Read the model definition and answer for the solid it produces. Units are mm, in the model's axes. A direction names the side the tool comes from. Coordinates: 2 decimals unless noted, no trailing zeros. Order: outer loops, then holes, each group sorted by start corner. A loop starts at its lowest first (then second) coordinate and runs counter-clockwise, first axis right, second up. Notation, with made-up numbers: (28, -4) -> (48, -4) arc R16 ccw to (48, 16) -> close; hole circle Ø6 at (1.5, -32). An arc over 180 degrees is marked (long way). Answer in a Markdown table with one row per item.
Autodesk Fusion 360 part; units mm, degrees
sketch "Sketch1" plane through (0, 0, 0) normal (0, 0, 1) x (1, 0, 0)
  line L0 (20, 20) -> (-20, 20)
  line L1 (-20, 20) -> (-20, -20)
  line L2 (-20, -20) -> (20, -20)
  line L3 (20, -20) -> (20, 20)
  line L4 (20, 20) -> (-20, -20) construction
  line L5 (-20, 20) -> (20, -20) construction
  dimension "d1" = 40
  dimension "d2" = 40
extrude "Extrude1" add sketch "Sketch1" along normal blind 8
sketch "Sketch2" plane through (0, 0, 8) normal (0, 0, 1) x (-1, 0, 0)
  line L0 (-20, 20) -> (-20, -20)
  line L1 (-20, -20) -> (20, -20)
  line L2 (20, -20) -> (20, 20)
  line L3 (20, 20) -> (-20, 20)
  circle A0 centre (15.5, -15.5) radius 1.6
  line L4 (-15.5, -15.5) -> (15.5, -15.5) construction
  line L5 (15.5, -15.5) -> (15.5, 15.5) construction
  line L6 (15.5, 15.5) -> (-15.5, 15.5) construction
  line L7 (-15.5, 15.5) -> (-15.5, -15.5) construction
  line L8 (-15.5, -15.5) -> (15.5, 15.5) construction
  line L9 (15.5, -15.5) -> (-15.5, 15.5) construction
  circle A1 centre (-15.5, 15.5) radius 1.6
  dimension "d5" = 3.2
  dimension "d6" = 31
  dimension "d7" = 31
  dimension "d8" = 3.2
extrude "Extrude2" cut sketch "Sketch2" against normal blind 15 contours A0 | A1
sketch "Sketch3" plane through (0, 0, 8) normal (0, 0, 1) x (-1, 0, 0)
  circle A0 centre (15.5, -15.5) radius 1.6
  circle A1 centre (-15.5, 15.5) radius 1.6
  line L0 (-20, 20) -> (-20, -20)
  line L1 (-20, -20) -> (20, -20)
  line L2 (20, -20) -> (20, 20)
  line L3 (20, 20) -> (-20, 20)
  line L4 (-17, -17) -> (17, -17) construction
  line L5 (17, -17) -> (17, 17) construction
  line L6 (17, 17) -> (-17, 17) construction
  line L7 (-17, 17) -> (-17, -17) construction
  line L8 (-17, -17) -> (17, 17) construction
  line L9 (17, -17) -> (-17, 17) construction
  circle A2 centre (-17, -17) radius 1.35
  circle A3 centre (17, 17) radius 1.35
  dimension "d11" = 34
  dimension "d12" = 34
  dimension "d13" = 2.7
  dimension "d14" = 2.7
extrude "Extrude3" cut sketch "Sketch3" against normal blind 12 contours A2 | A3
chamfer "Chamfer1" distance 1.8 angle 45 2 edges at (-14.0083, 14.9214, 8) (16.9917, -16.0786, 8)
chamfer "Chamfer2" distance 2 angle 45 4 edges at (20, -20, 4) (-20, -20, 4) (20, 20, 4) (-20, 20, 4)
sketch "Sketch4" plane through (0, 0, 8) normal (0, 0, 1) x (-1, 0, 0)
  circle A0 centre (15.5, -15.5) radius 3.4
  circle A1 centre (-17, -17) radius 1.35
  circle A2 centre (17, 17) radius 1.35
  line L0 (18, -20) -> (20, -18)
  line L1 (20, -18) -> (20, 18)
  line L2 (20, 18) -> (18, 20)
  line L3 (18, 20) -> (-18, 20)
  line L4 (-18, 20) -> (-20, 18)
  line L5 (-20, 18) -> (-20, -18)
  line L6 (-20, -18) -> (-18, -20)
  line L7 (-18, -20) -> (18, -20)
  circle A3 centre (-15.5, 15.5) radius 3.4
chamfer "Chamfer3" distance 0.5 angle 45 2 edges at (-15.7414, -17.4882, 8) (18.2586, 16.5118, 8)
sketch "Sketch5" plane through (0, 0, 8) normal (0, 0, 1) x (-1, 0, 0)
  line L0 (11, -20) -> (-11, -20)
  line L1 (-11, -20) -> (-11, -8)
  line L2 (-11, -8) -> (11, -8)
  line L3 (11, -8) -> (11, -20)
  line L4 (-18, -20) -> (18, -20)
  point P0 (0, -8)
  dimension "d20" = 22
  dimension "d21" = 12
extrude "Extrude4" cut sketch "Sketch5" against normal blind 15
fillet "Fillet1" radius 1 4 edges at (-11, 8, 4) (11, 8, 4) (11, 20, 4) (-11, 20, 4)
fillet "Fillet1" radius 1 8 edges at (-18, 20, 4) (-20, 18, 4) (-20, -18, 4) (-18, -20, 4) (18, -20, 4) (20, -18, 4) (20, 18, 4) (18, 20, 4)
chamfer "Chamfer4" distance 0.2 angle 45 1 faces at (-3.942, -7.6818, 0)
sketch "Sketch6" plane through (0, 0, 8) normal (0, 0, 1) x (-1, 0, 0)
  circle A0 centre (17, 17) radius 1.85
  circle A1 centre (15.5, -15.5) radius 3.4
  circle A2 centre (-15.5, 15.5) radius 3.4
  circle A3 centre (-17, -17) radius 1.85
  arc A4 (-18.2929, -19.7071) -> (-17.5858, -20) centre (-17.5858, -19) ccw
  line L0 (-17.5858, -20) -> (-12, -20)
  arc A5 (-12, -20) -> (-11, -19) centre (-12, -19) ccw
  line L1 (-11, -19) -> (-11, -9)
  arc A6 (-10, -8) -> (-11, -9) centre (-10, -9) ccw
  line L2 (-10, -8) -> (10, -8)
  arc A7 (11, -9) -> (10, -8) centre (10, -9) ccw
  line L3 (11, -9) -> (11, -19)
  arc A8 (11, -19) -> (12, -20) centre (12, -19) ccw
  line L4 (12, -20) -> (17.5858, -20)
  arc A9 (17.5858, -20) -> (18.2929, -19.7071) centre (17.5858, -19) ccw
  line L5 (18.2929, -19.7071) -> (19.7071, -18.2929)
  arc A10 (19.7071, -18.2929) -> (20, -17.5858) centre (19, -17.5858) ccw
  line L6 (20, -17.5858) -> (20, 17.5858)
  arc A11 (20, 17.5858) -> (19.7071, 18.2929) centre (19, 17.5858) ccw
  line L7 (19.7071, 18.2929) -> (18.2929, 19.7071)
  arc A12 (18.2929, 19.7071) -> (17.5858, 20) centre (17.5858, 19) ccw
  line L8 (17.5858, 20) -> (-17.5858, 20)
  arc A13 (-17.5858, 20) -> (-18.2929, 19.7071) centre (-17.5858, 19) ccw
  line L9 (-18.2929, 19.7071) -> (-19.7071, 18.2929)
  arc A14 (-19.7071, 18.2929) -> (-20, 17.5858) centre (-19, 17.5858) ccw
  line L10 (-20, 17.5858) -> (-20, -17.5858)
  arc A15 (-20, -17.5858) -> (-19.7071, -18.2929) centre (-19, -17.5858) ccw
  line L11 (-19.7071, -18.2929) -> (-18.2929, -19.7071)
  line L12 (-10, 20) -> (-10, 10)
  line L13 (-10, 10) -> (-20, 10)
  line L14 (-20, -10) -> (-11, -10)
  line L15 (0, -2.5) -> (0, -20)
  line L16 (10, 20) -> (10, 10)
  line L17 (10, 10) -> (20, 10)
  line L18 (20, -10) -> (11, -10)
  line L19 (11, -10) -> (10.0078, -10.7171)
  dimension "d29" = 10
  dimension "d32" = 10
  dimension "d37" = 10
extrude "Extrude5" cut sketch "Sketch6" against normal blind 2 contours L1 A6 L2 A7 L3 L6 L8 L10 L12 L13 L14 L16 L17 L18
fillet "Fillet2" radius 2 2 edges at (10, -10, 7) (-10, -10, 7)
Q1. The part is cut by section C-C (x = 2.5). Write down the section's boundary in (y, z).
Outcome:
| item | result |
|---|---|
| outline | (-20, 0.2) -> (-19.8, 0) -> (7.8, 0) -> (8, 0.2) -> (8, 6) -> (-20, 6) -> close |
Q2. Consider line 1 (Y direction, x = 14, z = 6.75); line 2 (Y direction, x = 15.5, z = 3.85); line 3 (X direction, y = 13, z = 6). Determine where each line is inside the solid, lowest interval first.
Outcome:
| item | result |
|---|---|
| line 1 | -20 to -17.04, -13.96 to -10, 10 to 20 |
| line 2 | -20 to -17.1, -13.9 to 20 |
| line 3 | -20 to -11, 11 to 20 |
Q3. The part is cut by section B-B (z = 7). Give the number of separate pieces and of enclosed holes in the cut face, then the cut area to 3 significant figures.
Outcome:
| item | result |
|---|---|
| separate pieces | 4 |
| enclosed holes | 4 |
| area | 322 mm² |
Q4. The part is cut by section D-D (y = -11.5). Write down the section's boundary in (x, z), then the cut area to 3 significant figures.
Outcome:
| item | result |
|---|---|
| outline | (-20, 0.2) -> (-19.8, 0) -> (19.8, 0) -> (20, 0.2) -> (20, 8) -> (10.06, 8) -> (10.06, 6) -> (-10.06, 6) -> (-10.06, 8) -> (-20, 8) -> close |
| area | 280 mm² |
Q5. For faces 1 (the face through (16.68, -16.58, 3.24)), 2 (the face through (12.7, -12.7, 8)), 3 (the face through (-10, -16, 7)), 4 (the face through (-16, -10, 7)), 5 (the face through (-11, 14, 4)), determine the directions among +Z, -Z, +X, -X, +Y, -Y from which every point of the face is accessible in a straight line to the end or side of a thin tool.
Outcome:
| item | result |
|---|---|
| face 1 | +Z, -Z |
| face 2 | +Z, +X, -X, +Y, -Y |
| face 3 | +Z, +Y, -Y |
| face 4 | +Z, +X, -X |
| face 5 | +Z, -Z, +Y |
Q6. For a pull along X with two mould halves and no side action, classify faces 6 (the face through (11.285, 19.699, 4.045)), 7 (the face through (19, -19, 4)), 8 (the face through (-19, 19, 4)) as pulls with the +X half, pulls with the -X half, needs draft (parallel to the pull), parting line crosses it, or undercut.
Outcome:
| item | result |
|---|---|
| face 6 | undercut |
| face 7 | pulls with the +X half |
| face 8 | pulls with the -X half |
Q7. Given pin 1 (2.5 mm diameter, centred on x = -15.5, y = 15.5, fed in from +Z); pin 2 (3 mm diameter, centred on x = -13.5, y = 4, fed in from +Z); pin 3 (2 mm diameter, centred on x = -5.5, z = 1, fed in from +Y); pin 4 (3.5 mm diameter, centred on x = 15.5, y = -15.5, fed in from +Z), each flat-ended and moving along its own axis, determine where each tip first touches the part or whether it passes through.
Outcome:
| item | result |
|---|---|
| pin 1 | through |
| pin 2 | z = 6 |
| pin 3 | y = 8 |
| pin 4 | z = 6.35 |
Q8. The part is cut by section A-A (z = 0.75). Write down the section's boundary in (x, y).
Outcome:
| item | result |
|---|---|
| outline | (-20, -17.59) arc R1 ccw to (-19.71, -18.29) -> (-18.29, -19.71) arc R1 ccw to (-17.59, -20) -> (17.59, -20) arc R1 ccw to (18.29, -19.71) -> (19.71, -18.29) arc R1 ccw to (20, -17.59) -> (20, 17.59) arc R1 ccw to (19.71, 18.29) -> (18.29, 19.71) arc R1 ccw to (17.59, 20) -> (12, 20) arc R1 ccw to (11, 19) -> (11, 9) arc R1 cw to (10, 8) -> (-10, 8) arc R1 cw to (-11, 9) -> (-11, 19) arc R1 ccw to (-12, 20) -> (-17.59, 20) arc R1 ccw to (-18.29, 19.71) -> (-19.71, 18.29) arc R1 ccw to (-20, 17.59) -> close; hole circle Ø2.7 at (-17, -17); hole circle Ø3.2 at (-15.5, 15.5); hole circle Ø3.2 at (15.5, -15.5); hole circle Ø2.7 at (17, 17) |
